from build123d import *

# Parameters (mm, degrees)
SKETCH1_W           = 30
SKETCH1_H           = 30.000023288
BOSS_EXTRUDE2_DEPTH = 32


with BuildPart() as part:
    # Sketch1 → Boss-Extrude2 (new body)
    with BuildSketch(Plane(origin=(0, 0, 0), x_dir=(1, 0, 0), z_dir=(0, 1, 0))):
        Polygon((-15, 15.000011644), (-15, -15.000011644), (-30, -0.01868994), align=None)
        Rectangle(SKETCH1_W, SKETCH1_H)
        Polygon((30, -0.01868994), (15, -15.000011644), (15, 15.000011644), align=None)
    extrude(amount=BOSS_EXTRUDE2_DEPTH)


solid = part.part
Verification items for the finished model (mm, model axes). Give positions to 0.01 mm unless a question says otherwise; leave off trailing zeros. Write each loop counter-clockwise with the first axis right and the second up, starting at its lowest first coordinate (ties: lowest second). Pieces come first, ordered by that corner, then holes. Notation, with made-up numbers: M 70,25.25 L 105,25.25 A8 cw 105,40.25 Z; hole C 74,48 d3. An arc over 180 degrees is marked long. Put each result on its own line as item: value. Start each with the question number.
1. Go/stop test with flat-tipped pins: pin 1 Ø10 at (y, z) = (27, 3) entering from +X; pin 2 Ø1 at (y, z) = (6.5, 3.5) entering from +X (3 decimals). Record where each tip stops, or that it passes through.
2. Section check C-C (x = -17.5). Record the cut outline in (y, z), and give its area (3 significant figures).
3. Section check A-A (y = 26). Record the cut outline in (x, z).
4. Scan lines: line 1 along Z through (x, y) = (-26.5, 2); line 2 along Z through (x, y) = (-17, 10); line 3 along X through (y, z) = (10.5, -2). Record each from-to range of solid material in increasing order. Write a range as [from, to].
5. Section check B-B (z = -9). Record the cut outline in (x, y), and give its area (3 significant figures).
Answer list:
1. pin 1: x = 30
1. pin 2: x = 27.015
2. outline: M 0,-12.5 L 32,-12.5 L 32,12.5 L 0,12.5 Z
2. area: 800 mm2
3. outline: M -30,0.02 L -15,-15 L 15,-15 L 30,0.02 L 15,15 L -15,15 Z
4. line 1: [-3.49, 3.51]
4. line 2: [-13, 13]
4. line 3: [-27.98, 27.98]
5. outline: M -20.99,0 L 20.99,0 L 20.99,32 L -20.99,32 Z
5. area: 1,340 mm2
